Part model, mm, in its own coordinate system. A direction names the side the tool comes from. Give positions to 0.01 mm unless a question says otherwise; leave off trailing zeros. Order: outer loops, then holes, each group sorted by start corner. A loop starts at its lowest first (then second) coordinate and runs counter-clockwise, first axis right, second up. Notation, with made-up numbers: M 11.25,54 L 38.25,54 A13 cw 38.25,79 Z; hole C 34.25,85.5 d2. An arc over 180 degrees is marked long. One line per question, with ' | ' between items.
```python
from build123d import *

# Parameters (mm, degrees)
F0_R     = 5
F1_DEPTH = 8
F2_R     = 2
F3_R     = 0.5
F4_DEPTH = 205
F6_DEPTH = 10


with BuildPart() as f1:
    # F0 (on Front) → F1 (new body)
    with BuildSketch(Plane.XZ):
        Polygon((-25, 50), (-25, -20), (40, -20), (40, 80), (-260, 80), (-260, -20), (-230, -20), (-230, 50), align=None)
        Circle(F0_R, mode=Mode.SUBTRACT)
    extrude(amount=F1_DEPTH)

    # F2
    f2_edges = [f1.edges().sort_by_distance(p)[0] for p in [
        (-260, -8, 30),
        (-245, -8, -20),
        (-230, -8, 15),
        (-127.5, -8, 50),
        (-25, -8, 15),
        (7.5, -8, -20),
        (40, -8, 30),
        (-110, -8, 80),
        (-260, -4, 80),
        (-260, -4, -20),
        (40, -4, 80),
        (40, -4, -20),
        (-25, -4, -20),
        (-25, -4, 50),
        (-230, -4, 50),
        (-230, -4, -20),
        (-245, 0, -20),
        (-230, 0, 15),
        (-127.5, 0, 50),
        (7.5, 0, -20),
        (40, 0, 30),
        (-110, 0, 80),
        (-260, 0, 30),
        (-25, 0, 15),
    ]]
    fillet(f2_edges, radius=F2_R)

    # F3 (on face) → F4 (join, through all)
    with BuildSketch(Plane(origin=(-25, 0, 0), x_dir=(0, -1, 0), z_dir=(-1, 0, 0))):
        with Locations((4, 0)):
            Circle(F3_R)
    extrude(amount=F4_DEPTH)

    # F5 (on face) → F6 (join)
    with BuildSketch(Plane.XZ.offset(8)):
        with BuildLine():
            ThreePointArc((-235.3830339919, 11.7465816491), (-242.2588387865, 24.1047088707), (-254.6169660081, 17.2289040761))
            Line((-254.6169660081, 17.2289040761), (-283.3303219183, -83.5077349835))
            Line((-283.3303219183, -83.5077349835), (-286.420911747, -130.8315102833))
            Line((-286.420911747, -130.8315102833), (-264.096389902, -88.9900574105))
            Line((-264.096389902, -88.9900574105), (-235.3830339919, 11.7465816491))
        make_face()
    extrude(amount=F6_DEPTH)


solid = f1.part
```
1. Slice it at A-A on x = -69.5. Give the cut face in (y, z).
Worked out:
outline: M -8,52 A2 ccw -6,50 L -2,50 A2 ccw 0,52 L 0,78 A2 ccw -2,80 L -6,80 A2 ccw -8,78 Z; C -4,0 d1
2. Slice it at B-B on x = 0. Give the cut face in (y, z).
Worked out:
outline: M -8,-18 A2 ccw -6,-20 L -2,-20 A2 ccw 0,-18 L 0,-5 L -8,-5 Z; M -8,5 L 0,5 L 0,78 A2 ccw -2,80 L -6,80 A2 ccw -8,78 Z
3. Slice it at D-D on z = -112. Give the cut face in (x, y), then the cut area to 3 significant figures.
Worked out:
outline: M -285.19,-18 L -276.37,-18 L -276.37,-8 L -285.19,-8 Z | area: 88.2 mm2
4. Drop flat-ended pins along their axis: pin 1 (2 mm diameter, centred on x = -239.5, y = -4.5, fed in from -Z); pin 2 (1.2 mm diameter, centred on y = -4, z = 24, fed in from -X); pin 3 (3 mm diameter, centred on x = -112.5, y = -4.5, fed in from -Z). Give the stop position or say it passes through.
Worked out:
pin 1: stops at z = -20 | pin 2: stops at x = -260 | pin 3: stops at z = -0.5
5. Slice it at C-C on y = -12.75. Give the cut face in (x, z).
Worked out:
outline: M -286.42,-130.83 L -264.1,-88.99 L -235.38,11.75 A10 ccw -254.62,17.23 L -283.33,-83.51 Z
6. Mould opens along X. For faces 1 (the cylindrical face through (-1.08, -3.94, -4.88)), 2 (the cylindrical face through (-242.048, -12.93, 24.042)), 3 (the flat face through (-275.415, -12.93, -110.204)), 4 (the flat face through (-112, 0, 63)) say: released by +X, released by -X, zero draft, split by the parting line, or undercut.
Worked out:
face 1: undercut | face 2: split by the parting line | face 3: released by +X | face 4: zero draft
7. Probe L1, parallel to X at y = -5.25, z = -17.5; L2, parallel to Z at x = 0, y = -3.5; L3, parallel to Z at x = -250.5, y = -6. List the from-to ranges inside material, lowest first. Write a range as from..to.
Worked out:
L1: x = -260..-230, -25..40 | L2: z = -20..-5, 5..80 | L3: z = -20..80
8. Tool access for faces 5 (the flat face through (-268.77, -12.93, -32.43)), 6 (the flat face through (-284.854, -12.93, -106.838)), 7 (the flat face through (-249.94, -12.93, -39.33)): list every direction of +Z, -Z, +X, -X, +Y, -Y with a clear straight run to the whole face (end or side of a thin tool).
Worked out:
face 5: +Z, -X, -Y | face 6: +Z, -X, +Y, -Y | face 7: -Z, +X, -Y
